from build123d import *

# Parameters (mm, degrees)
SKETCH1_R           = 15
SKETCH1_R_2         = 10
BOSS_EXTRUDE1_DEPTH = 6


with BuildPart() as part:
    # Sketch1 → Boss-Extrude1 (new body)
    with BuildSketch(Plane(origin=(0, 0, 0), x_dir=(1, 0, 0), z_dir=(0, 1, 0))):
        Polygon((0, 0), (19, 0), (19, -6), (29, -6), (29, 0), (65, 0), (65, -6), (75, -6), (75, 0), (94, 0), (94, 106), (75, 106), (75, 112), (65, 112), (65, 106), (29, 106), (29, 112), (19, 112), (19, 106), (0, 106), align=None)
        with Locations(Location((25, 53, 0), (0, 0, 270))):
            Circle(SKETCH1_R, mode=Mode.SUBTRACT)
        with Locations(Location((69, 53, 0), (0, 0, 270))):
            Circle(SKETCH1_R, mode=Mode.SUBTRACT)
        with Locations(Location((47, 81, 0), (0, 0, 270))):
            Circle(SKETCH1_R, mode=Mode.SUBTRACT)
        with Locations(Location((47, 25, 0), (0, 0, 270))):
            Circle(SKETCH1_R, mode=Mode.SUBTRACT)
        with Locations(Location((20, 20, 0), (0, 0, 270))):
            Circle(SKETCH1_R_2, mode=Mode.SUBTRACT)
        with Locations(Location((20, 86, 0), (0, 0, 270))):
            Circle(SKETCH1_R_2, mode=Mode.SUBTRACT)
        with Locations(Location((74, 86, 0), (0, 0, 270))):
            Circle(SKETCH1_R_2, mode=Mode.SUBTRACT)
        with Locations(Location((74, 20, 0), (0, 0, 270))):
            Circle(SKETCH1_R_2, mode=Mode.SUBTRACT)
    extrude(amount=BOSS_EXTRUDE1_DEPTH)


solid = part.part
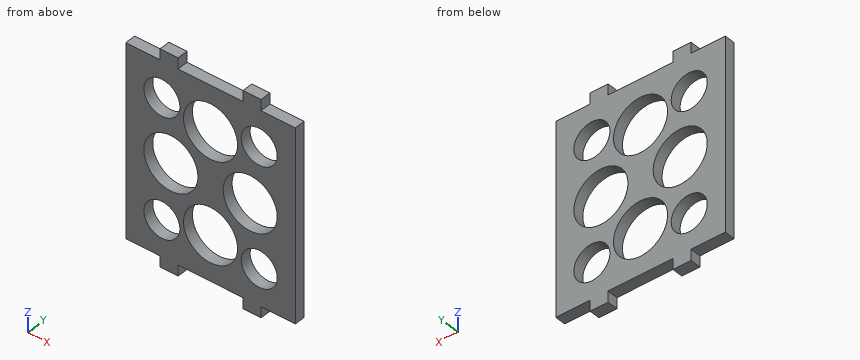
Read the model definition and answer for the solid it produces. Units are mm, in the model's axes. Round coordinates to 2 decimals unless told otherwise and drop trailing zeros. Order: outer loops, then holes, each group sorted by start corner. A loop starts at its lowest first (then second) coordinate and runs counter-clockwise, first axis right, second up. Notation, with made-up numbers: (47.5, 81.25) - (51.5, 81.25) arc R35 ccw to (51.5, 113.25) - close; hole circle Ø5 at (52.25, 79.5). An arc over 180 degrees is marked (long way). Use one line per item in the form item = value. Start each with the question number.
(1) The part is cut by section C-C (y = 2.55). Count the separate pieces of the cut face and the enclosed holes in it, then the cut area to 3 significant figures.
(2) Find the intervals of material crossed by line 1 along X through (y, z) = (4.1, -60); line 2 along X through (y, z) = (2.9, -86); line 3 along X through (y, z) = (3.35, -43.5), in increasing order. Write a range as from..to.
(3) The part is cut by section B-B (x = 76.5). Give the vertices of the cut face in (y, z).
(4) The part is cut by section D-D (z = -94). Give the vertices of the cut face in (x, y).
(5) The part is cut by section A-A (z = -53). Give the vertices of the cut face in (x, y), then the cut area to 3 significant figures.
(6) Flat-ended cylindrical pins translate along their axes: pin 1 Ø1.8 at (x, y) = (10, 4) entering from -Z; pin 2 Ø24 at (x, z) = (47, -81) entering from -Y; pin 3 Ø1.8 at (y, z) = (3, -108) entering from +X; pin 4 Ø3 at (x, y) = (5, 3.5) entering from +Z. Find the tip coordinate at first contact, or state that the pin passes through.
Checked values:
q1.separate_pieces = 1
q1.enclosed_holes = 8
q1.area = 6,120 mm^2
q2.line_1 = 0..11.73, 38.27..55.73, 82.27..94
q2.line_2 = 0..10, 30..32.86, 61.14..64, 84..94
q2.line_3 = 0..13.39, 36.61..57.39, 80.61..94
q3.outline = (0, -106) - (6, -106) - (6, -95.68) - (0, -95.68) - close; (0, -76.32) - (6, -76.32) - (6, -65.99) - (0, -65.99) - close; (0, -40.01) - (6, -40.01) - (6, -29.68) - (0, -29.68) - close; (0, -10.32) - (6, -10.32) - (6, 0) - (0, 0) - close
q4.outline = (0, 0) - (14, 0) - (14, 6) - (0, 6) - close; (26, 0) - (39.52, 0) - (39.52, 6) - (26, 6) - close; (54.48, 0) - (68, 0) - (68, 6) - (54.48, 6) - close; (80, 0) - (94, 0) - (94, 6) - (80, 6) - close
q5.outline = (0, 0) - (10, 0) - (10, 6) - (0, 6) - close; (40, 0) - (54, 0) - (54, 6) - (40, 6) - close; (84, 0) - (94, 0) - (94, 6) - (84, 6) - close
q5.area = 204 mm^2
q6.pin_1 = -106
q6.pin_2 = through
q6.pin_3 = 75
q6.pin_4 = 0
